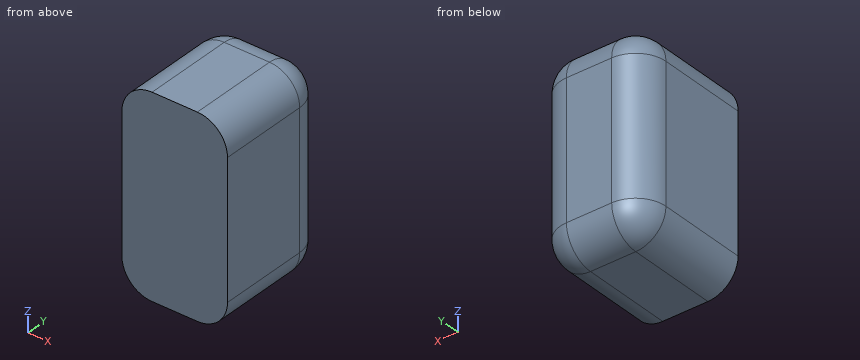
```python
from build123d import *

# Parameters (mm, degrees)
SKETCH1_W           = 16.51
SKETCH1_H           = 10.16
BOSS_EXTRUDE1_DEPTH = 4.445
FILLET1_R           = 2.54


with BuildPart() as part:
    # Sketch1 → Boss-Extrude1 (new body, symmetric)
    with BuildSketch(Plane(origin=(0, 0, 0), x_dir=(0, 0, -1), z_dir=(1, 0, 0))):
        with Locations((8.255, 5.08)):
            Rectangle(SKETCH1_W, SKETCH1_H)
    extrude(amount=BOSS_EXTRUDE1_DEPTH, both=True)

    # Fillet1
    fillet1_edges = [part.edges().sort_by_distance(p)[0] for p in [
        (4.445, 5.08, -16.51),
        (4.445, 10.16, -8.255),
        (4.445, 5.08, 0),
        (-4.445, 10.16, -8.255),
        (-4.445, 5.08, -16.51),
        (-4.445, 5.08, 0),
        (0, 10.16, 0),
        (0, 10.16, -16.51),
    ]]
    fillet(fillet1_edges, radius=FILLET1_R)


solid = part.part
```
Could you check a few things on this model? Use its own coordinates, in mm. Coordinates: 2 decimals unless noted, no trailing zeros. Order: outer loops, then holes, each group sorted by start corner. A loop starts at its lowest first (then second) coordinate and runs counter-clockwise, first axis right, second up. Notation, with made-up numbers: M 46.5,40 L 89.5,40 A35 ccw 89.5,76 Z; hole C 64,-8 d2. An arc over 180 degrees is marked long. Use one line per item in the form item = value. Start each with the question number.
1. Suppose I cut it at A-A on x = -1.25. Write out the boundary of the cut face in (y, z).
2. Suppose I cut it at D-D on y = 8.75. Write out the boundary of the cut face in (x, z) (3 decimals).
3. Suppose I cut it at B-B on y = 2.75. Write out the boundary of the cut face in (x, z) (3 decimals).
4. Suppose I cut it at C-C on z = -5. Write out the boundary of the cut face in (x, y) (3 decimals), then the cut area to 3 significant figures.
5. Please list where these lines run through material, in increasing order: line 1 (Z direction, x = 2, y = 3); line 2 (X direction, y = 7.75, z = -4); line 3 (Y direction, x = 2.5, z = -11.5).
Geometry says:
q1.outline = M 0,-16.51 L 7.62,-16.51 A2.54 ccw 10.16,-13.97 L 10.16,-2.54 A2.54 ccw 7.62,0 L 0,0 Z
q2.outline = M -4.18,-13.97 A2.275 ccw -1.905,-16.245 L 1.905,-16.245 A2.275 ccw 4.18,-13.97 L 4.18,-2.54 A2.275 ccw 1.905,-0.265 L -1.905,-0.265 A2.275 ccw -4.18,-2.54 Z
q3.outline = M -4.445,-13.97 A2.54 ccw -1.905,-16.51 L 1.905,-16.51 A2.54 ccw 4.445,-13.97 L 4.445,-2.54 A2.54 ccw 1.905,0 L -1.905,0 A2.54 ccw -4.445,-2.54 Z
q4.outline = M -4.445,0 L 4.445,0 L 4.445,7.62 A2.54 ccw 1.905,10.16 L -1.905,10.16 A2.54 ccw -4.445,7.62 Z
q4.area = 87.6 mm^2
q5.line_1 = -16.51 to 0
q5.line_2 = -4.44 to 4.44
q5.line_3 = 0 to 10.09
